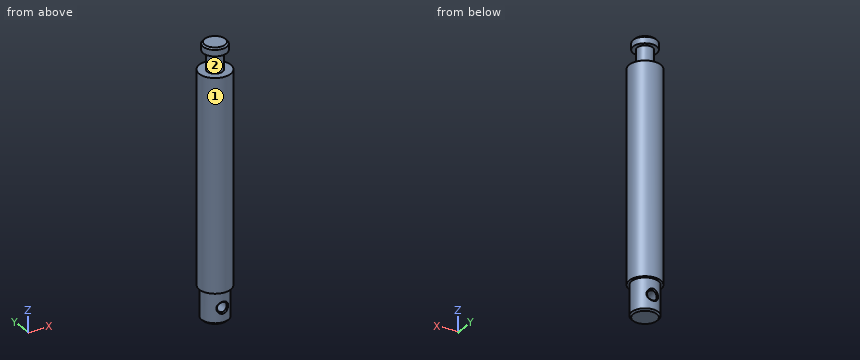
Autodesk Inventor part; units mm, degrees
ref_plane "YZ Plane" through (0, 0, 0) normal (1, 0, 0) x (0, 1, 0)
ref_plane "XZ Plane" through (0, 0, 0) normal (0, 1, 0) x (-1, 0, 0)
ref_plane "XY Plane" through (0, 0, 0) normal (0, 0, 1) x (1, 0, 0)
sketch "Sketch1" plane through (0, 0, 0) normal (1, 0, 0) x (0, 1, 0)
  line L0 (0, 0) -> (0, -170)
  line L1 (0, 0) -> (6.5, 0)
  line L2 (6.5, 0) -> (7.5, -1)
  line L3 (7.5, -1) -> (7.5, -5)
  line L4 (7.5, -5) -> (5, -5)
  line L5 (5, -5) -> (5, -17)
  line L6 (5, -17) -> (10, -17)
  line L7 (10, -17) -> (10, -150)
  line L8 (10, -150) -> (8.5, -150)
  line L9 (8.5, -150) -> (8.5, -169)
  line L10 (7.5, -170) -> (0, -170)
  line L11 (8.5, -169) -> (7.5, -170)
  point P0 (8.5, -170)
  dimension "d0" = 170
  dimension "d1" = 17
  dimension "d2" = 20
  dimension "d3" = 10
  dimension "d4" = 15
  dimension "d5" = 5
  dimension "d6" = 1
  dimension "d7" = 1
  dimension "d8" = 12
  dimension "d9" = 20
  dimension "d10" = 1
  dimension "d11" = 1
revolve "Revolution1" add sketch "Sketch1" angle 360 about axis through (0, 0, 0) along (0, 0, -1)
sketch "Sketch2" plane through (0, 0, 0) normal (0, 1, 0) x (-1, 0, 0)
  circle A0 centre (0, -160) radius 3
  line L0 (-7.5, -170) -> (7.5, -170)
  point P0 (0, 0)
  dimension "d13" = 6
  dimension "d14" = 10
extrude "Extrusion1" cut sketch "Sketch2" along normal through all both and the other way through all
chamfer "Chamfer1" distance 0.75 angle 45 4 edges at (3, 7.953, -159.9995) (-2.2741, 8.1902, -158.0433) (-2.2734, 8.1903, -161.9575) (3, -7.953, -160.0011)
thread "Thread1"
Check sheet for the modelled part. Datum: model origin and axes. Units: mm. Face numbers are marked on the shaded views. Round coordinates to 2 decimals unless told otherwise and drop trailing zeros. Loops run counter-clockwise (first coordinate to the right, second up) from the corner with the lowest first, then second, coordinate; pieces in that order, holes last. Notation, with made-up numbers: (2.25, 46) -> (30.25, 46) arc R12 ccw to (30.25, 59) -> close; hole circle Ø7 at (30.25, 28.5). An arc over 180 degrees is marked (long way). Write item = value, one per line. Start each with the question number.
1) Gauge pin test, flat ends, axial feed: pin 1 Ø5 at (x, z) = (0, -160) entering from +Y; pin 2 Ø5 at (y, z) = (4, -69) entering from -X; pin 3 Ø1.5 at (x, z) = (-1.5, -32.5) entering from +Y; pin 4 Ø2 at (y, z) = (6, -69.5) entering from -X. Record the tip position at first contact, or that the pin passes through.
2) Sectioned sample at A-A, the plane y = 0. Record the cut outline in (x, z), plus the area to 3 significant figures.
3) Thickness scan on probe 1 along Z at (x, y) = (0, -3.75); probe 2 along X at (y, z) = (-4, -160); probe 3 along X at (y, z) = (-0.75, -160). Record the ranges inside material, lowest first.
4) Sectioned sample at B-B, the plane z = -59. Record the cut outline in (x, y).
5) Release check for a two-part mould opening along Z. For the marked faces 1 and 2 record: released by +Z, released by -Z, zero draft, split by the parting line, or undercut.
Results are:
q1.pin_1 = through
q1.pin_2 = -9.89
q1.pin_3 = 9.97
q1.pin_4 = -8.66
q2.outline = (-10, -150) -> (-8.5, -150) -> (-8.5, -169) -> (-7.5, -170) -> (7.5, -170) -> (8.5, -169) -> (8.5, -150) -> (10, -150) -> (10, -17) -> (5, -17) -> (5, -5) -> (7.5, -5) -> (7.5, -1) -> (6.5, 0) -> (-6.5, 0) -> (-7.5, -1) -> (-7.5, -5) -> (-5, -5) -> (-5, -17) -> (-10, -17) -> close; hole circle Ø6 at (0, -160)
q2.area = 3,160 mm^2
q3.probe_1 = -170 to -163, -157 to 0
q3.probe_2 = -7.5 to -3, 3 to 7.5
q3.probe_3 = -8.47 to -3, 3 to 8.47
q4.outline = circle Ø20 at (0, 0)
q5.face_1 = zero draft
q5.face_2 = undercut
